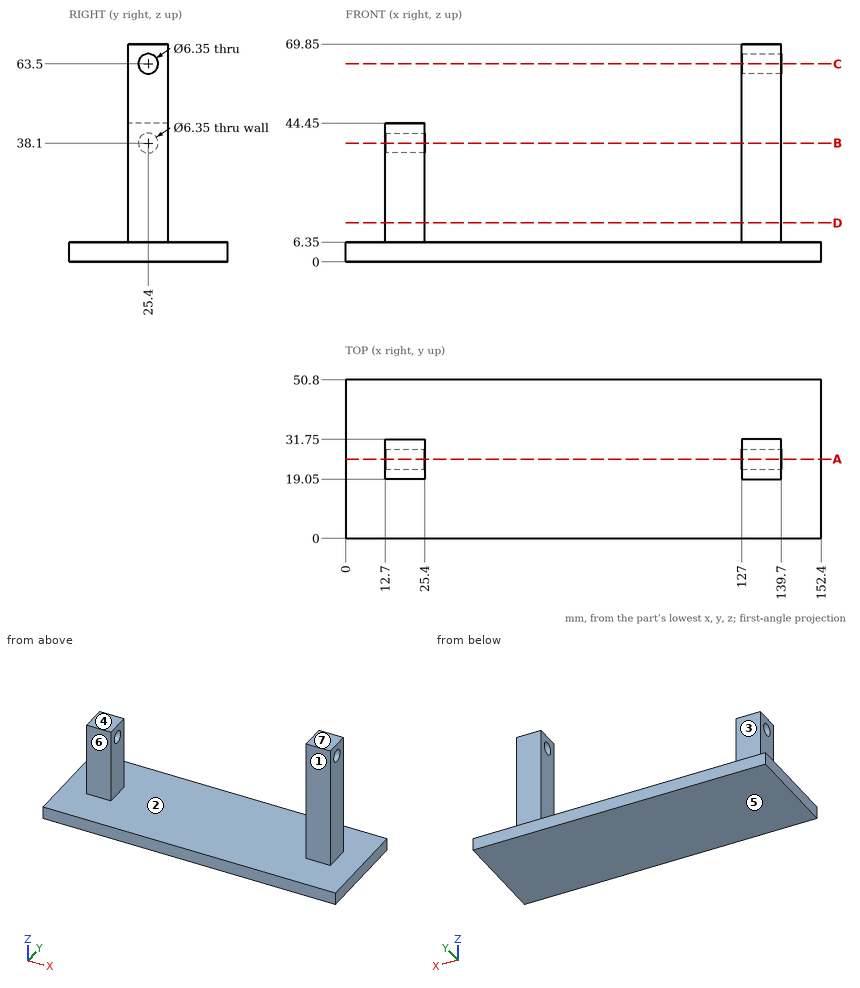
Verification items for this drawing (mm, ordinates from the low corner). A direction names the side the tool comes from. Coordinates: 2 decimals unless noted, no trailing zeros. Write each loop counter-clockwise with the first axis right and the second up, starting at its lowest first coordinate (ties: lowest second). Pieces come first, ordered by that corner, then holes. Notation, with made-up numbers: M 89,32.5 L 93,32.5 A6 ccw 93,41.5 Z; hole C -10,48.25 d4. An arc over 180 degrees is marked long. Answer as a JSON object with one key per item and string values.
1. Section check A-A, the plane y = 25.4. Enter the section's corners in (x, z) (3 decimals).
Answers below:
{"outline": "M 0,0 L 152.4,0 L 152.4,6.35 L 139.7,6.35 L 139.7,60.325 L 127,60.325 L 127,6.35 L 25.4,6.35 L 25.4,34.925 L 12.7,34.925 L 12.7,6.35 L 0,6.35 Z; M 12.7,41.275 L 25.4,41.275 L 25.4,44.45 L 12.7,44.45 Z; M 127,66.675 L 139.7,66.675 L 139.7,69.85 L 127,69.85 Z"}
2. Section check C-C, the plane z = 63.5. Enter the section's corners in (x, y) (3 decimals), plus the area to 3 significant figures.
Answers below:
{"outline": "M 127,19.05 L 139.7,19.05 L 139.7,22.225 L 127,22.225 Z; M 127,28.575 L 139.7,28.575 L 139.7,31.75 L 127,31.75 Z", "area": "80.6 mm²"}
3. Section check D-D, the plane z = 12.5. Enter the section's corners in (x, y), plus the area to 3 significant figures.
Answers below:
{"outline": "M 12.7,19.05 L 25.4,19.05 L 25.4,31.75 L 12.7,31.75 Z; M 127,19.05 L 139.7,19.05 L 139.7,31.75 L 127,31.75 Z", "area": "323 mm²"}
4. Tool access check on the marked faces 3, 4, 5, 6 and 7. Record the directions out of +Z, -Z, +X, -X, +Y, -Y that give a thin tool (end or side, any length) a straight path to the whole face; none if there is none.
Answers below:
{"face 3": "+Z, +X, -X, +Y", "face 4": "+Z, -X, +Y, -Y", "face 5": "-Z, +X, -X, +Y, -Y", "face 6": "+Z, +X, -X, -Y", "face 7": "+Z, +X, -X, +Y, -Y"}
5. Section check B-B, the plane z = 38.1. Enter the section's corners in (x, y) (3 decimals), plus the area to 3 significant figures.
Answers below:
{"outline": "M 12.7,19.05 L 25.4,19.05 L 25.4,22.225 L 12.7,22.225 Z; M 12.7,28.575 L 25.4,28.575 L 25.4,31.75 L 12.7,31.75 Z; M 127,19.05 L 139.7,19.05 L 139.7,31.75 L 127,31.75 Z", "area": "242 mm²"}
6. Scan lines: L1, parallel to Z at x = 132, y = 25; L2, parallel to Y at x = 20.25, z = 38.1 (3 decimals); L3, parallel to X at y = 24, z = 18. Record each from-to range of solid material in increasing order.
Answers below:
{"L1": "z = 0 to 60.35, 66.65 to 69.85", "L2": "y = 19.05 to 22.225, 28.575 to 31.75", "L3": "x = 12.7 to 25.4, 127 to 139.7"}
7. Draft check along X on the marked faces 1 and 2. Enter one of: released by +X, released by -X, zero draft, split by the parting line, or undercut.
Answers below:
{"face 1": "zero draft", "face 2": "undercut"}
8. Go/stop test with flat-tipped pins: pin 1 Ø6.5 at (y, z) = (26, 29.5) entering from +X; pin 2 Ø2 at (x, z) = (132.5, 18) entering from +Y; pin 3 Ø14 at (y, z) = (23, 29.5) entering from -X; pin 4 Ø12 at (y, z) = (40, 48) entering from +X. Record where each tip stops, or that it passes through.
Answers below:
{"pin 1": "stops at x = 139.7", "pin 2": "stops at y = 31.75", "pin 3": "stops at x = 12.7", "pin 4": "passes through"}
